```python
from build123d import *

# Parameters (mm, degrees)
SALIENTE_EXTRUIR1_DEPTH = 50.8
CROQUIS4_R              = 6.35
CORTAR_EXTRUIR4_DEPTH   = 50.8
REDONDEO1_R             = 2.54
CROQUIS7_R              = 6.35
CORTAR_EXTRUIR5_DEPTH   = 3.175


with BuildPart() as part:
    # Croquis3 → Saliente-Extruir1 (new body)
    with BuildSketch(Plane.XY):
        Polygon((0, 0), (0, 76.2), (38.1, 76.2), (38.1, 0), (41.275, 0), (41.275, 79.375), (-3.175, 79.375), (-3.175, 0), align=None)
    extrude(amount=SALIENTE_EXTRUIR1_DEPTH)

    # Croquis4 → Cortar-Extruir4 (cut)
    with BuildSketch(Plane(origin=(41.275, 0, 0), x_dir=(0, 0, -1), z_dir=(1, 0, 0))):
        with BuildLine():
            Line((-50.8, 0), (-38.099999933, 0))
            ThreePointArc((-38.099999933, 0), (-47.080256097, 3.719743855), (-50.8, 12.7))
            Line((-50.8, 12.7), (-50.8, 0))
        make_face()
        with Locations((-38.1, 12.7)):
            Circle(CROQUIS4_R)
        with BuildLine():
            Line((0, 0), (0, 79.375))
            Line((0, 79.375), (-26.18309853, 8.309389636))
            ThreePointArc((-26.18309853, 8.309389636), (-30.836073748, 2.282448685), (-38.099999933, 0))
            Line((-38.099999933, 0), (0, 0))
        make_face()
    extrude(amount=-CORTAR_EXTRUIR4_DEPTH, mode=Mode.SUBTRACT)

    # Redondeo1
    redondeo1_edges = [part.edges().sort_by_distance(p)[0] for p in [
        (-3.175, 79.375, 25.4),
        (41.275, 79.375, 25.4),
    ]]
    fillet(redondeo1_edges, radius=REDONDEO1_R)

    # Croquis7 → Cortar-Extruir5 (cut)
    with BuildSketch(Plane(origin=(0, 79.375, 0), x_dir=(1, 0, 0), z_dir=(0, 1, 0))):
        with Locations((19.05, -25.4)):
            Circle(CROQUIS7_R)
    extrude(amount=-CORTAR_EXTRUIR5_DEPTH, mode=Mode.SUBTRACT)


solid = part.part
```
Verification items for the finished model (mm, model axes). A direction names the side the tool comes from. Round coordinates to 2 decimals unless told otherwise and drop trailing zeros. Write each loop counter-clockwise with the first axis right and the second up, starting at its lowest first coordinate (ties: lowest second). Pieces come first, ordered by that corner, then holes.
1. Section check D-D on z = 8. Enter the section's corners in (x, y) (3 decimals), plus the area to 3 significant figures.
2. Draft check along X on faces 1 (the cylindrical face through (24.916, 77.81, 27.832)), 2 (the flat face through (-0.6, 49.27, 11.09)), 3 (the cylindrical face through (40.55, 78.61, 25.76)), 4 (the flat face through (23, 76.2, 20)). Enter one of: +X half, -X half, draft (parallel to the pull), parting line (faces both ways), or undercut.
3. Section check A-A on x = 19.05. Enter the section's corners in (y, z) (3 decimals).
4. Section check B-B on y = 44.5. Enter the section's corners in (x, z) (3 decimals).
5. Section check C-C on z = 30.5. Enter the section's corners in (x, y) (3 decimals), plus the area to 3 significant figures.
6. Gauge pin test, flat ends, axial feed: P1, Ø1, axis at x = 32, z = 22.5, coming from the -Y side; P2, Ø14.5, axis at y = 12.7, z = 38.1, coming from the +X side (3 decimals). Record the tip position at first contact, or that the pin passes through.
7. Access from +Z, -Z, +X, -X, +Y, -Y to the whole of each face (thin tool, end or side, straight path). Record for faces 5 (the flat face through (-3.175, 47, 31)), 6 (the flat face through (38.1, 47, 31)).
8. Scan lines: L1, parallel to X at y = 26, z = 24 (3 decimals); L2, parallel to Y at x = 26, z = 14.5 (3 decimals); L3, parallel to Y at x = -2, z = 38. Record each from-to range of solid material in increasing order.
Answer:
1. outline: (-3.175, 57.662) - (0, 57.662) - (0, 76.2) - (38.1, 76.2) - (38.1, 57.662) - (41.275, 57.662) - (41.275, 76.835) arc R2.54 ccw to (38.735, 79.375) - (-0.635, 79.375) arc R2.54 ccw to (-3.175, 76.835) - close
1. area: 256 mm2
2. face 1: undercut
2. face 2: draft
2. face 3: +X half
2. face 4: undercut
3. outline: (76.2, 1.17) - (79.375, 0) - (79.375, 19.05) - (76.2, 19.05) - close; (76.2, 31.75) - (79.375, 31.75) - (79.375, 50.8) - (76.2, 50.8) - close
4. outline: (-3.175, 12.849) - (0, 12.849) - (0, 50.8) - (-3.175, 50.8) - close; (38.1, 12.849) - (41.275, 12.849) - (41.275, 50.8) - (38.1, 50.8) - close
5. outline: (-3.175, 2.525) - (0, 2.525) - (0, 76.2) - (15.267, 76.2) - (15.267, 79.375) - (-0.635, 79.375) arc R2.54 ccw to (-3.175, 76.835) - close; (22.833, 76.2) - (38.1, 76.2) - (38.1, 2.525) - (41.275, 2.525) - (41.275, 76.835) arc R2.54 ccw to (38.735, 79.375) - (22.833, 79.375) - close
5. area: 582 mm2
6. P1: stops at y = 76.2
6. P2: stops at x = 41.275
7. face 5: +Z, -Z, -X, +Y, -Y
7. face 6: +Z, -Z, -Y
8. L1: x = -3.175 to 0, 38.1 to 41.275
8. L2: y = 76.2 to 79.375
8. L3: y = 0 to 6.35, 19.05 to 78.98
